```python
from build123d import *

# Parameters (mm, degrees)
F1_DEPTH = 63.5
F2_DEPTH = 25.4
F3_DEPTH = 15.875
F5_R     = 6.35


with BuildPart() as f1:
    # F0 (on Front) → F1 (new body, symmetric)
    with BuildSketch(Plane.XZ):
        Polygon((-41.275, -9.525), (41.275, -9.525), (41.275, 9.525), (22.098, 9.525), (-41.275, 9.525), align=None)
    extrude(amount=F1_DEPTH, both=True)

    # F0 (on Front) → F2 (join, symmetric)
    with BuildSketch(Plane.XZ):
        with BuildLine():
            Line((22.098, 9.525), (41.275, 9.525))
            Line((41.275, 9.525), (41.275, 27.0002))
            ThreePointArc((41.275, 27.0002), (45.9246798487, 38.2255201513), (57.15, 42.8752))
            Line((57.15, 42.8752), (60.325, 42.8752))
            Line((60.325, 42.8752), (60.325, 62.0522))
            Line((60.325, 62.0522), (57.15, 62.0522))
            ThreePointArc((57.15, 62.0522), (32.3644931058, 51.7857068942), (22.098, 27.0002))
            Line((22.098, 27.0002), (22.098, 9.525))
        make_face()
        Polygon((60.325, 66.675), (60.325, 62.0522), (60.325, 42.8752), (60.325, 38.1), (85.725, 38.1), (85.6915154391, 66.675), align=None)
    extrude(amount=F2_DEPTH, both=True)

    # F0 (on Front) → F3 (join)
    with BuildSketch(Plane.XZ):
        with BuildLine():
            add(Edge.make_bspline(
                [(-41.275, 9.525), (-39.1135952527, 29.6751279876), (8.2365749404, 64.628906548), (57.15, 62.0522)],
                knots=[0, 0, 0, 0, 111.5642745902, 111.5642745902, 111.5642745902, 111.5642745902], degree=3))
            Line((-41.275, 9.525), (22.098, 9.525))
            Line((22.098, 9.525), (22.098, 27.0002))
            ThreePointArc((22.098, 27.0002), (32.3644931058, 51.7857068942), (57.15, 62.0522))
        make_face()
    extrude(amount=F3_DEPTH)

    # F0 (on Front) → F4 (revolve)
    with BuildSketch(Plane.XZ):
        Polygon((111.125, 66.675), (85.6915154391, 66.675), (85.725, 38.1), (111.125, 38.1), align=None)
    revolve(axis=Axis((85.7082577195, 0, 52.3875), (-0.0011718124, 0, 0.9999993134)))

    # F5
    f5_edges = [f1.edges().sort_by_distance(p)[0] for p in [
        (-41.275, -63.5, 0),
        (41.275, -63.5, 0),
        (41.275, 63.5, 0),
        (-41.275, 63.5, 0),
    ]]
    fillet(f5_edges, radius=F5_R)


solid = f1.part
```
The model under review builds one solid part; all positions refer to its coordinate system, in mm. A direction names the side the tool comes from. Round coordinates to 2 decimals unless told otherwise and drop trailing zeros. Loops run counter-clockwise (first coordinate to the right, second up) from the corner with the lowest first, then second, coordinate; pieces in that order, holes last. Notation, with made-up numbers: M -4,-24.5 L 47,-24.5 A28 cw 47,-1.5 Z; hole C 51,53 d1. An arc over 180 degrees is marked long. Write item = value, one per line.
Item 1: Take a section at A-A on z = 6. Write out the cut boundary in (x, y) (3 decimals), then the cut area to 3 significant figures.
Return value:
outline = M -41.275,-57.15 A6.35 ccw -34.925,-63.5 L 34.925,-63.5 A6.35 ccw 41.275,-57.15 L 41.275,57.15 A6.35 ccw 34.925,63.5 L -34.925,63.5 A6.35 ccw -41.275,57.15 Z
area = 10,400 mm2
Item 2: Insertion check: P1, Ø20.5, axis at x = 70.5, y = -14, coming from the -Z side; P2, Ø5, axis at y = 9.5, z = 20.5, coming from the -X side; P3, Ø3, axis at x = 35.5, z = 26, coming from the +Y side. Each pin has a flat end and moves straight along its axis. Give the tip position at first contact, or say it passes through.
Return value:
P1 = 38.04
P2 = 22.1
P3 = 25.4
Item 3: Machinability: for faces 3 (the flat face through (22.098, -21, 18)), 4 (the cylindrical face through (32.64, 12.52, 52.06)), which of the approach directions +Z, -Z, +X, -X, +Y, -Y give a long, thin tool a straight path to every point of the face, cutting with its end or side? Answer none if there is none.
Return value:
face_3 = +Z, -X, -Y
face_4 = +Z, -X, +Y
Item 4: The part is to be moulded in two halves that separate along X. For faces 1 (the cylindrical face through (32.64, -20.7, 52.06)), 2 (the flat face through (60.325, 13, 41)), say which applies: released by +X, released by -X, zero draft, split by the parting line, or undercut.
Return value:
face_1 = released by -X
face_2 = undercut
Item 5: Take a section at B-B on y = 33.5. Write out the cut boundary in (x, z) (3 decimals), then the cut area to 3 significant figures.
Return value:
outline = M -41.275,-9.525 L 41.275,-9.525 L 41.275,9.525 L -41.275,9.525 Z
area = 1,570 mm2
Item 6: For line 1 (Z direction, x = -25, y = 50.5) (3 decimals); line 2 (X direction, y = 12.5, z = 19.5) (3 decimals); line 3 (X direction, y = 55, z = 9) (3 decimals), list the stretches that pass through material, from the lowest coordinate up. Write a range as [from, to].
Return value:
line_1 = [-9.525, 9.525]
line_2 = [22.098, 41.275]
line_3 = [-41.275, 41.275]
